The model under review builds one solid part; all positions refer to its coordinate system, in mm. Face numbers are marked on the shaded views. A direction names the side the tool comes from. Give positions to 0.01 mm unless a question says otherwise; leave off trailing zeros. Order: outer loops, then holes, each group sorted by start corner. A loop starts at its lowest first (then second) coordinate and runs counter-clockwise, first axis right, second up. Notation, with made-up numbers: (28.25, -2) -> (43.25, -2) arc R26 cw to (43.25, 13) -> close; hole circle Ø9 at (29, 83.25). An arc over 180 degrees is marked (long way). Use one line per item in the form item = value.
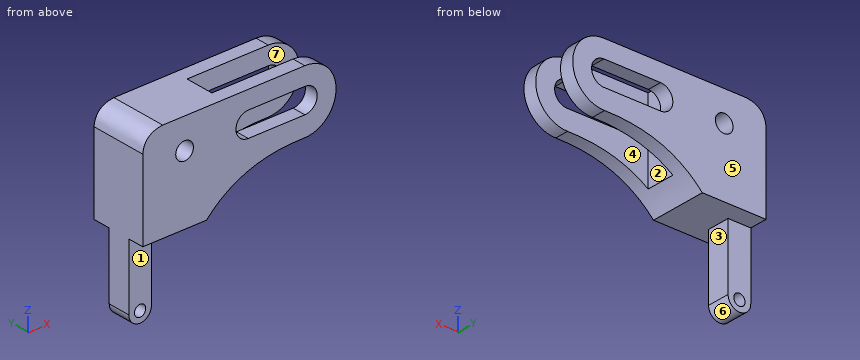
```python
from build123d import *

# Parameters (mm, degrees)
SKETCH1_R           = 6.25
BOSS_EXTRUDE1_DEPTH = 40
SKETCH3_W           = 16
SKETCH3_H           = 16
BOSS_EXTRUDE2_DEPTH = 55
SKETCH4_W           = 79.487617275
SKETCH4_H           = 20.321855451
CUT_EXTRUDE1_DEPTH  = 60.08
CUT_EXTRUDE2_DEPTH  = 60.08
SKETCH8_R           = 4
CUT_EXTRUDE3_DEPTH  = 60.08


with BuildPart() as part:
    # Sketch1 → Boss-Extrude1 (new body)
    with BuildSketch(Plane(origin=(0, 0, 0), x_dir=(1, 0, 0), z_dir=(0, 1, 0))):
        with BuildLine():
            Line((-45, 0), (0, 0))
            add(Edge.make_bspline(
                [(0, 0), (17.365983088, -18.556062235), (40.507326339, -25.876534392), (69.05598636, -25.291140997)],
                knots=[0, 0, 0, 0, 1, 1, 1, 1], degree=3))
            ThreePointArc((69.05598636, -25.291140997), (91.549113489, -47.102951703), (69.507873161, -69.371305461))
            Line((69.507873161, -69.371305461), (-19.337413001, -69.371305461))
            Line((-19.337413001, -69.371305461), (-30.918760516, -69.371305461))
            add(Edge.make_bspline(
                [(-45, -56.695680455), (-43.898759302, -68.233062502), (-30.918760516, -69.371305461)],
                knots=[0, 0, 0, 1, 1, 1], degree=2))
            Line((-45, -56.695680455), (-45, -50.496042729))
            Line((-45, -50.496042729), (-45, 0))
        make_face()
        with Locations(Location((-15.478366003, -48, 0), (0, 0, 270))):
            Circle(SKETCH1_R, mode=Mode.SUBTRACT)
        with BuildLine():
            Line((29.521633997, -39.304319545), (69.521633997, -39.304319545))
            ThreePointArc((69.521633997, -39.304319545), (78.217314452, -48), (69.521633997, -56.695680455))
            Line((69.521633997, -56.695680455), (29.521633997, -56.695680455))
            ThreePointArc((29.521633997, -56.695680455), (20.825953542, -48), (29.521633997, -39.304319545))
        make_face(mode=Mode.SUBTRACT)
    extrude(amount=BOSS_EXTRUDE1_DEPTH)

    # Sketch3 → Boss-Extrude2 (add)
    with BuildSketch(Plane(origin=(0, 0, 0), x_dir=(-1, 0, 0), z_dir=(0, 0, -1))):
        with Locations((37, 19.479254529)):
            Rectangle(SKETCH3_W, SKETCH3_H)
    extrude(amount=BOSS_EXTRUDE2_DEPTH)

    # Sketch4 → Cut-Extrude1 (cut)
    with BuildSketch(Plane.XY.offset(69.371305461)):
        with Locations((51.911602749, 19.849304399)):
            Rectangle(SKETCH4_W, SKETCH4_H)
    extrude(amount=-CUT_EXTRUDE1_DEPTH, mode=Mode.SUBTRACT)

    # Sketch7 → Cut-Extrude2 (cut)
    with BuildSketch(Plane(origin=(0, 27.479254529, 0), x_dir=(1, 0, 0), z_dir=(0, 1, 0))):
        with BuildLine():
            Line((-45, 46.438944543), (-45, 55))
            Line((-45, 55), (-29, 55))
            Line((-29, 55), (-29, 46.438944543))
            ThreePointArc((-29, 46.438944543), (-37, 54.438944543), (-45, 46.438944543))
        make_face()
    extrude(amount=-CUT_EXTRUDE2_DEPTH, mode=Mode.SUBTRACT)

    # Sketch8 → Cut-Extrude3 (cut)
    with BuildSketch(Plane(origin=(0, 27.479254529, 0), x_dir=(1, 0, 0), z_dir=(0, 1, 0))):
        with Locations(Location((-37, 46.819480791, 0), (0, 0, 180))):
            Circle(SKETCH8_R)
    extrude(amount=-CUT_EXTRUDE3_DEPTH, mode=Mode.SUBTRACT)


solid = part.part
```
1. Tool access review of the marked faces 1, 2 and 3: name each direction out of +Z, -Z, +X, -X, +Y, -Y from which nothing blocks a thin tool from reaching the whole face with its end or side.
Values:
face_1 = -Z, +X, -X, -Y
face_2 = +Z, -Z, +X
face_3 = -Z, +X, +Y, -Y
2. Add section B-B on z = 28. Give the boundary of the cut face in (x, y).
Values:
outline = (-45, 0) -> (80.1, 0) -> (80.1, 9.69) -> (12.17, 9.69) -> (12.17, 30.01) -> (80.1, 30.01) -> (80.1, 40) -> (-45, 40) -> close
3. For pin 1 Ø4 at (y, z) = (32.5, 14) entering from +X; pin 2 Ø10 at (y, z) = (15.5, 41) entering from +X; pin 3 Ø13 at (x, z) = (-35, -14.5) entering from -Y, all flat-tipped, find the tip position at first contact; note any pin that passes through.
Values:
pin_1 = 21.33
pin_2 = 12.17
pin_3 = 11.48
4. Add section C-C on x = 40. Count the separate pieces of the cut face and the enclosed holes in it, then the cut area to 3 significant figures.
Values:
separate_pieces = 4
enclosed_holes = 0
area = 578 mm^2
5. For L1, parallel to X at y = 9, z = 48; L2, parallel to X at y = 23.5, z = 48; L3, parallel to Y at x = 81, z = 57.5, list the stretches that pass through material, from the lowest coordinate up.
Values:
L1 = -45 to -21.73, -9.23 to 20.83, 78.22 to 91.54
L2 = -45 to -21.73, -9.23 to 12.17
L3 = 0 to 9.69, 30.01 to 40
6. Add section A-A on z = 46.5. Give the boundary of the cut face in (x, y).
Values:
outline = (-45, 0) -> (-21.55, 0) -> (-21.55, 40) -> (-45, 40) -> close; (-9.41, 0) -> (20.96, 0) -> (20.96, 9.69) -> (12.17, 9.69) -> (12.17, 30.01) -> (20.96, 30.01) -> (20.96, 40) -> (-9.41, 40) -> close; (78.09, 0) -> (91.53, 0) -> (91.53, 9.69) -> (78.09, 9.69) -> close; (78.09, 30.01) -> (91.53, 30.01) -> (91.53, 40) -> (78.09, 40) -> close
7. The part is to be moulded in two halves that separate along Y. For the marked faces 4, 5, 6 and 7, say which applies: +Y half, -Y half, draft (parallel to the pull), parting line (faces both ways), or undercut.
Values:
face_4 = undercut
face_5 = +Y half
face_6 = draft
face_7 = undercut
